Check sheet for the modelled part. Datum: model origin and axes. Units: mm. A direction names the side the tool comes from. Round coordinates to 2 decimals unless told otherwise and drop trailing zeros. Loops run counter-clockwise (first coordinate to the right, second up) from the corner with the lowest first, then second, coordinate; pieces in that order, holes last. Notation, with made-up numbers: (86, -17.5) - (92, -17.5) arc R11 cw to (92, 0.5) - close; hole circle Ø1 at (57.5, 2.5). An arc over 180 degrees is marked (long way). Return JSON: item names as keys, results as strings.
from build123d import *

# Parameters (mm, degrees)
SKETCH_1_W          = 15
SKETCH_1_H          = 15
SKETCH_1_W_2        = 12
SKETCH_1_H_2        = 12
EXTRUDE_1_DEPTH     = 740
SKETCH_2_R          = 2
CUT_EXTRUDE_1_DEPTH = 741.190009389
SKETCH_3_R          = 2
CUT_EXTRUDE_2_DEPTH = 741.190009389


with BuildPart() as part:
    # ｽｹｯﾁ1 → 押し出し-薄板1 (new body)
    with BuildSketch(Plane(origin=(0, 0, 0), x_dir=(1, 0, 0), z_dir=(0, 1, 0))):
        Rectangle(SKETCH_1_W, SKETCH_1_H)
        Rectangle(SKETCH_1_W_2, SKETCH_1_H_2, mode=Mode.SUBTRACT)
    extrude(amount=EXTRUDE_1_DEPTH)

    # ｽｹｯﾁ2 → ｶｯﾄ - 押し出し1 (cut, through all)
    with BuildSketch(Plane(origin=(7.5, 0, 0), x_dir=(0, 0, -1), z_dir=(1, 0, 0))):
        with Locations((0, 50)):
            Circle(SKETCH_2_R)
        with Locations((0, 10)):
            Circle(SKETCH_2_R)
        with Locations((0, 715)):
            Circle(SKETCH_2_R)
        with Locations((0, 705)):
            Circle(SKETCH_2_R)
        with Locations((0, 505)):
            Circle(SKETCH_2_R)
        with Locations((0, 495)):
            Circle(SKETCH_2_R)
    extrude(amount=-CUT_EXTRUDE_1_DEPTH, mode=Mode.SUBTRACT)

    # ｽｹｯﾁ3 → ｶｯﾄ - 押し出し2 (cut, through all)
    with BuildSketch(Plane.XY.offset(7.5)):
        with Locations((0, 735)):
            Circle(SKETCH_3_R)
        with Locations((0, 725)):
            Circle(SKETCH_3_R)
    extrude(amount=-CUT_EXTRUDE_2_DEPTH, mode=Mode.SUBTRACT)


solid = part.part
Q1. Draft check along X on faces 1 (the face through (0, 365, 7.5)), 2 (the face through (0, 365, 6)), 3 (the face through (7.5, 365, 0)). Enter one of: released by +X, released by -X, zero draft, split by the parting line, or undercut.
Answer key:
{"face 1": "zero draft", "face 2": "undercut", "face 3": "released by +X"}
Q2. Sectioned sample at A-A (y = 601). Enter the section's corners in (x, z), plus the area to 3 significant figures.
Answer key:
{"outline": "(-7.5, -7.5) - (7.5, -7.5) - (7.5, 7.5) - (-7.5, 7.5) - close; hole (-6, -6) - (6, -6) - (6, 6) - (-6, 6) - close", "area": "81.0 mm²"}
Q3. Depth check by flat-ended pin: P1, Ø3.5, axis at y = 495, z = 0, coming from the +X side. Enter the tip coordinate at first touch or a pass-through.
Answer key:
{"P1": "passes through"}
Q4. Tool access check on faces 4 (the face through (6, 365, 0)), 5 (the face through (-7, 0, 0)). Record the directions out of +Z, -Z, +X, -X, +Y, -Y that give a thin tool (end or side, any length) a straight path to the whole face; none if there is none.
Answer key:
{"face 4": "+Y, -Y", "face 5": "+Z, -Z, +X, -X, -Y"}
Q5. Scan lines: probe 1 along X at (y, z) = (725, 6.8); probe 2 along X at (y, z) = (530.5, 0.75). Record each from-to range of solid material in increasing order. Write a range as [from, to].
Answer key:
{"probe 1": "x = [-7.5, -2], [2, 7.5]", "probe 2": "x = [-7.5, -6], [6, 7.5]"}
